```python
from build123d import *

# Parameters (mm, degrees)
F0_R     = 209.55
F0_R_2   = 15.875
F1_DEPTH = 55.626
F2_R     = 130.175
F2_R_2   = 101.6
F3_DEPTH = 6.35
F4_R     = 2.54


with BuildPart() as f1:
    # F0 (on Front) → F1 (new body)
    with BuildSketch(Plane.XZ):
        Circle(F0_R)
        with Locations((-123.478522, -123.478522)):
            Circle(F0_R_2, mode=Mode.SUBTRACT)
        with Locations((-45.196276, -168.674797)):
            Circle(F0_R_2, mode=Mode.SUBTRACT)
        with Locations((-168.674797, -45.196276)):
            Circle(F0_R_2, mode=Mode.SUBTRACT)
        with Locations((45.196276, -168.674797)):
            Circle(F0_R_2, mode=Mode.SUBTRACT)
        with Locations((123.478522, -123.478522)):
            Circle(F0_R_2, mode=Mode.SUBTRACT)
        with Locations((168.674797, -45.196276)):
            Circle(F0_R_2, mode=Mode.SUBTRACT)
        with Locations((-168.674797, 45.196276)):
            Circle(F0_R_2, mode=Mode.SUBTRACT)
        with Locations((-123.478522, 123.478522)):
            Circle(F0_R_2, mode=Mode.SUBTRACT)
        with Locations((-45.196276, 168.674797)):
            Circle(F0_R_2, mode=Mode.SUBTRACT)
        with Locations((168.674797, 45.196276)):
            Circle(F0_R_2, mode=Mode.SUBTRACT)
        with Locations((45.196276, 168.674797)):
            Circle(F0_R_2, mode=Mode.SUBTRACT)
        with Locations((123.478522, 123.478522)):
            Circle(F0_R_2, mode=Mode.SUBTRACT)
    extrude(amount=F1_DEPTH)

    # F2 (on face) → F3 (join)
    with BuildSketch(Plane.XZ.offset(55.626)):
        Circle(F2_R)
        Circle(F2_R_2, mode=Mode.SUBTRACT)
    extrude(amount=F3_DEPTH)

    # F4
    f4_edges = [f1.edges().sort_by_distance(p)[0] for p in [
        (-209.55, -55.626, 0),
        (-209.55, 0, 0),
        (-130.175, -61.976, 0),
        (-130.175, -55.626, 0),
    ]]
    fillet(f4_edges, radius=F4_R)


solid = f1.part
```
Part model, mm, in its own coordinate system. A direction names the side the tool comes from. Round coordinates to 2 decimals unless told otherwise and drop trailing zeros. Loops run counter-clockwise (first coordinate to the right, second up) from the corner with the lowest first, then second, coordinate; pieces in that order, holes last. Notation, with made-up numbers: (-6.75, -27) -> (5.25, -27) arc R16 cw to (5.25, -3) -> close; hole circle Ø3 at (-1.75, 52.5). An arc over 180 degrees is marked (long way). Use CSV: the item, a comma, the result in double quotes. Start each with the question number.
1) Cut at B-B, the plane y = -40. Give the number of separate pieces and of enclosed holes in the cut face, plus the area to 3 significant figures.
2) Which spindle directions (+Z, -Z, +X, -X, +Y, -Y) get a long thin tool onto all of the face, cutting with end or side? Do faces 5 (the cylindrical face through (-125.545, -27.424, 139.218)), 6 (the flat face through (-95, -55.626, 95)). Say none if no direction does.
3) Cut at A-A, the plane z = 0. Write the cut outline in (x, y) (3 decimals).
4) Cut at C-C, the plane x = 0. Write the cut outline in (y, z) (3 decimals), plus the area to 3 significant figures.
5) Wall check: L1, parallel to X at y = -41, z = 111.5; L2, parallel to Z at x = -46, y = -41.5; L3, parallel to Z at x = -49.5, y = -37. Give the ranges that are in metal, low to high. Write a range as [from, to].
6) Pull direction X, two halves, no side cores. Call faces 1 (the cylindrical face through (121.41, -27.42, 139.22)), 2 (the cylindrical face through (-47.263, -27.424, 184.415)), 3 (the flat face through (-86, -61.976, -56)), 4 (the cylindrical face through (-103.3, -58.79, -79.21)): +X half, -X half, draft (parallel to the pull), parting line (faces both ways), or undercut.
7) Drop flat-ended pins along their axis: P1, Ø1.5, axis at x = -48.5, z = 127.5, coming from the -Y side; P2, Ø10, axis at y = -46.5, z = -68, coming from the +X side; P3, Ø5, axis at x = -68, y = -21, coming from the +Z side; P4, Ø12, axis at x = 94, z = -138.5, coming from the +Y side. Give the stop position or say it passes through.
Determined:
1,separate pieces,"1"
1,enclosed holes,"12"
1,area,"128,000 mm2"
2,face 5,"+Y, -Y"
2,face 6,"-Y"
3,outline,"(-209.55, -53.086) arc R2.54 ccw to (-207.01, -55.626) -> (-132.715, -55.626) arc R2.54 cw to (-130.175, -58.166) -> (-130.175, -59.436) arc R2.54 ccw to (-127.635, -61.976) -> (-101.6, -61.976) -> (-101.6, -55.626) -> (101.6, -55.626) -> (101.6, -61.976) -> (127.635, -61.976) arc R2.54 ccw to (130.175, -59.436) -> (130.175, -58.166) arc R2.54 cw to (132.715, -55.626) -> (207.01, -55.626) arc R2.54 ccw to (209.55, -53.086) -> (209.55, -2.54) arc R2.54 ccw to (207.01, 0) -> (-207.01, 0) arc R2.54 ccw to (-209.55, -2.54) -> close"
4,outline,"(-61.976, -127.635) arc R2.54 ccw to (-59.436, -130.175) -> (-58.166, -130.175) arc R2.54 cw to (-55.626, -132.715) -> (-55.626, -207.01) arc R2.54 ccw to (-53.086, -209.55) -> (-2.54, -209.55) arc R2.54 ccw to (0, -207.01) -> (0, 207.01) arc R2.54 ccw to (-2.54, 209.55) -> (-53.086, 209.55) arc R2.54 ccw to (-55.626, 207.01) -> (-55.626, 132.715) arc R2.54 cw to (-58.166, 130.175) -> (-59.436, 130.175) arc R2.54 ccw to (-61.976, 127.635) -> (-61.976, 101.6) -> (-55.626, 101.6) -> (-55.626, -101.6) -> (-61.976, -101.6) -> close"
4,area,"23,700 mm2"
5,L1,"x = [-177.42, -133.9], [-113.06, 113.06], [133.9, 177.42]"
5,L2,"z = [-204.44, -184.53], [-152.82, 152.82], [184.53, 204.44]"
5,L3,"z = [-203.62, -183.96], [-153.39, 153.39], [183.96, 203.62]"
6,face 1,"undercut"
6,face 2,"undercut"
6,face 3,"draft"
6,face 4,"parting line"
7,P1,"stops at y = -55.63"
7,P2,"stops at x = 199.86"
7,P3,"stops at z = 199.05"
7,P4,"stops at y = 0"
